The model under review builds one solid part; all positions refer to its coordinate system, in mm. A direction names the side the tool comes from. Coordinates: 2 decimals unless noted, no trailing zeros. Write each loop counter-clockwise with the first axis right and the second up, starting at its lowest first coordinate (ties: lowest second). Pieces come first, ordered by that corner, then holes. Notation, with made-up numbers: (-30, 80) - (29, 80) arc R19 ccw to (29, 93) - close; hole circle Ø4 at (-31.5, 0.25). An arc over 180 degrees is marked (long way). Return JSON: item names as keys, results as strings. Group by question number.
(1) Draft analysis for pull direction X (two halves, no side actions). For faces 5 (the face through (-1, 1, 0)), 6 (the face through (-57.909, -16, 59)), 7 (the face through (-68.354, -1, 21)), state which applies: released by +X, released by -X, zero draft, split by the parting line, or undercut.
(2) We need section A-A on z = 71. State the section outline as (x, y) points, then the cut area to 3 significant figures.
(3) Tool access review of faces 1 (the face through (63.205, 0.411, 30.258)), 2 (the face through (31.107, 37, 64)), 3 (the face through (-20.635, 37, 64)), 4 (the face through (-1, 0, 12.7)): name each direction out of +Z, -Z, +X, -X, +Y, -Y from which nothing blocks a thin tool from reaching the whole face with its end or side.
(4) We need section D-D on x = -44. State the section outline as (y, z) points.
(5) For pin 1 Ø5 at (x, y) = (6.5, -36.5) entering from +Z; pin 2 Ø8 at (x, y) = (45, 10.5) entering from +Z, all flat-tipped, find the tip position at first contact; note any pin that passes through.
(6) To check wall thickness, follow L1, parallel to X at y = 4, z = 69.5; L2, parallel to Y at x = -46.5, z = 73.5; L3, parallel to Z at x = -64.25, y = 0. State the ranges of each line that lie inside material, in increasing order. Write a range as from..to.
(7) We need section B-B on y = -17.5. State the section outline as (x, z) points, then the cut area to 3 significant figures.
(8) We need section C-C on y = -31. State the section outline as (x, z) points, then the cut area to 3 significant figures.
```python
from build123d import *

# Parameters (mm, degrees)
F0_W      = 136.7070674896
F0_H      = 81.1290219426
F1_DEPTH  = 76.2
F2_W      = 115.8186718822
F2_H      = 68.073771894
F3_DEPTH  = 63.5
F4_W      = 51.7421588302
F4_H      = 6.5276250243
F5_DEPTH  = 25.4
F6_W      = 53.3207450062
F6_H      = 6.5276250243
F7_DEPTH  = 25.4
F8_R      = 19.5019980074
F9_DEPTH  = 25.4
F10_R     = 16.2167518515
F11_DEPTH = 25.4


with BuildPart() as f1:
    # F0 (on Top) → F1 (new body)
    with BuildSketch(Plane.XY):
        Rectangle(F0_W, F0_H)
    extrude(amount=F1_DEPTH)

    # F2 (on face) → F3 (cut)
    with BuildSketch(Plane.XY.offset(76.2)):
        Rectangle(F2_W, F2_H)
    extrude(amount=-F3_DEPTH, mode=Mode.SUBTRACT)

    # F4 (on face) → F5 (cut)
    with BuildSketch(Plane.XY.offset(76.2)):
        with Locations((5.2360128611, 37.3006984591)):
            Rectangle(F4_W, F4_H)
    extrude(amount=-F5_DEPTH, mode=Mode.SUBTRACT)

    # F6 (on face) → F7 (cut)
    with BuildSketch(Plane.XY.offset(76.2)):
        with Locations((3.2774237916, -37.3006984591)):
            Rectangle(F6_W, F6_H)
    extrude(amount=-F7_DEPTH, mode=Mode.SUBTRACT)

    # F8 (on face) → F9 (cut)
    with BuildSketch(Plane(origin=(-68.3535337448, 0, 0), x_dir=(0, -1, 0), z_dir=(-1, 0, 0))):
        with Locations((0, 42.4992851913)):
            Circle(F8_R)
    extrude(amount=-F9_DEPTH, mode=Mode.SUBTRACT)

    # F10 (on face) → F11 (cut)
    with BuildSketch(Plane.YZ.offset(68.3535337448)):
        with Locations((-7.0724547841, 44.6449071169)):
            Circle(F10_R)
    extrude(amount=-F11_DEPTH, mode=Mode.SUBTRACT)


solid = f1.part
```
Ans:
{
 "1": {"face 5": "zero draft", "face 6": "undercut", "face 7": "released by -X"},
 "2": {"outline": "(-68.35, -40.56) - (-23.38, -40.56) - (-23.38, -34.04) - (-57.91, -34.04) - (-57.91, 34.04) - (-20.64, 34.04) - (-20.64, 40.56) - (-68.35, 40.56) - close; (29.94, -40.56) - (68.35, -40.56) - (68.35, 40.56) - (31.11, 40.56) - (31.11, 34.04) - (57.91, 34.04) - (57.91, -34.04) - (29.94, -34.04) - close", "area": "2,520 mm²"},
 "3": {"face 1": "+X", "face 2": "+Z, +Y", "face 3": "+Z, +Y, -Y", "face 4": "+Z"},
 "4": {"outline": "(-40.56, 0) - (40.56, 0) - (40.56, 76.2) - (34.04, 76.2) - (34.04, 12.7) - (-34.04, 12.7) - (-34.04, 76.2) - (-40.56, 76.2) - close"},
 "5": {"pin 1": "z = 50.8", "pin 2": "z = 12.7"},
 "6": {"L1": "-68.35..-57.91, 57.91..68.35", "L2": "-40.56..-34.04, 34.04..40.56", "L3": "0..23, 62..76.2"},
 "7": {"outline": "(-68.35, 0) - (68.35, 0) - (68.35, 32.23) - (57.91, 32.23) - (57.91, 12.7) - (-57.91, 12.7) - (-57.91, 33.89) - (-68.35, 33.89) - close; (-68.35, 51.11) - (-57.91, 51.11) - (-57.91, 76.2) - (-68.35, 76.2) - close; (57.91, 57.06) - (68.35, 57.06) - (68.35, 76.2) - (57.91, 76.2) - close", "area": "2,620 mm²"},
 "8": {"outline": "(-68.35, 0) - (68.35, 0) - (68.35, 76.2) - (57.91, 76.2) - (57.91, 12.7) - (-57.91, 12.7) - (-57.91, 76.2) - (-68.35, 76.2) - close", "area": "3,060 mm²"}
}
